Autodesk Inventor part; units mm, degrees
ref_plane "Work Plane1" through (29, 0, 0) normal (0, -1, 0) x (1, 0, 0)
ref_plane "YZ Plane" through (0, 0, 0) normal (1, 0, 0) x (0, 1, 0)
ref_plane "XZ Plane" through (0, 0, 0) normal (0, 1, 0) x (-1, 0, 0)
sketch "Sketch1" plane through (0, 0, 0) normal (0, 0, 1) x (1, 0, 0)
  line L0 (-1.1667, 0) -> (80, 0)
  line L1 (80, 0) -> (80, 2.5)
  line L2 (80, 2.5) -> (58, 2.5)
  line L3 (58, 2.5) -> (57.5091, 2.5)
  line L4 (57.5091, 2.5) -> (0, 2.5)
  line L5 (0, 2.5) -> (0, 4.25)
  line L6 (0, 4.25) -> (-5, 4.25)
  line L7 (-5, 4.25) -> (-5, 2.3094)
  line L8 (-5, 2.3094) -> (-2.5, 2.3094)
  line L9 (-2.5, 2.3094) -> (-1.1667, 0)
  line L10 (-16, 0) -> (61, 0)
  line L11 (0, -0.85) -> (0, 5.1)
  line L12 (58, 2.5) -> (0, 2.5) construction
  dimension "d1" = 22
  dimension "d2" = 0.4909
  dimension "d3" = 5
  dimension "d4" = 2.5
  dimension "d5" = 60
  dimension "d6" = 5
  dimension "d7" = 5
  dimension "d8" = 4.6188
  dimension "d9" = 8.5
  dimension "d26" = 80
revolve "Body" add sketch "Sketch1" angle 360 about axis through (-1.1667, 0, 0) along (1, 0, 0)
sketch "Sketch2" plane through (-5, 0, 0) normal (-1, 0, 0) x (0, 0, 1)
  circle A0 centre (0, 0) radius 2.3094
  line L0 (0, -5.95) -> (0, 5.95)
  line L1 (-5.95, 0) -> (5.95, 0)
  line L2 (2.3094, 0) -> (1.1547, -2)
  line L3 (1.1547, -2) -> (-1.1547, -2)
  line L4 (-1.1547, -2) -> (-2.3094, 0)
  line L5 (-2.3094, 0) -> (-1.1547, 2)
  line L6 (-1.1547, 2) -> (1.1547, 2)
  line L7 (1.1547, 2) -> (2.3094, 0)
extrude "Slot" add sketch "Sketch2" against normal up to next contours L7 A0 | A0 L2 | L6 L0 A0 | A0 L0 L3 | L0 L6 A0 | A0 L3 L0 | L4 A0 | A0 L5
fillet "Fillet1" radius 0.5 1 edges at (-5, -4.25, 0)
thread "Thread"
chamfer "Chamfer1" distance 0.4908 distance2 0.4908 1 edges at (80, -2.5, 0) measured on face at (80, 0.2278, 0.5045)
ref_plane "Work Plane1" through (29, 0, 0) normal (0, -1, 0) x (1, 0, 0)
fillet "Fillet2" radius 0.2 1 edges at (0, -2.5, 0)
equation "\"d30\" = R"
equation "\"d17\" = RR"
equation "\"d13\" = GEL"
equation "\"d15\" = -0.5 * SPD + 0.5 * GD"
equation "\"d16\" = GUL"
equation "\"d1\" = GEL"
equation "\"d3\" = KOH"
equation "\"d4\" = INTI"
equation "\"d6\" = GD"
equation "\"d7\" = BDM"
equation "\"d8\" = 1.1547 * SW"
equation "\"d9\" = KOD"
equation "\"d26\" = NLG"
equation "\"GD\" = NND"
equation "\"NLG\" = 80"
equation "\"GEL\" = 22"
equation "\"KOD\" = 8.5"
equation "\"KOH\" = 5"
equation "\"INTI\" = 2.5"
equation "\"GAL\" = 0.61345 * PTC"
equation "\"GUL\" = 0.61345 * PTC"
equation "\"BDM\" = NND"
equation "\"SW\" = 4"
equation "\"RR\" = 0.5"
equation "\"SPD\" = NND - 1.2269 * PTC"
equation "\"R\" = 0.2"
equation "\"TOA\" = 30deg"
equation "\"GD1\" = THREADDIA - 1.2269 * PTC"
equation "\"THREADDIA\" = 5"
equation "\"FAWI\" = 45deg"
equation "\"ANG\" = 120deg"
equation "\"PTC\" = 0.8"
equation "\"NND\" = 5"
equation "\"E0\" = 1.155 * SW"
properties material "Steel, Mild"
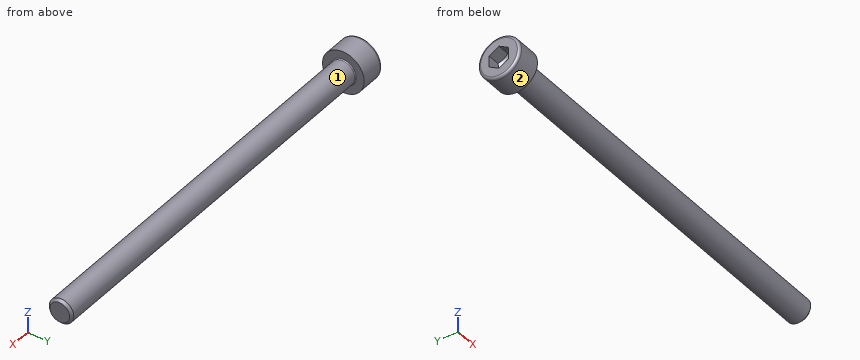
The listing builds one solid part. Answer for the finished solid, in the listing's coordinates (mm). Face numbers are marked on the shaded views. A direction names the side the tool comes from. Give positions to 0.01 mm unless a question says otherwise; leave off trailing zeros. Write each loop counter-clockwise with the first axis right and the second up, starting at its lowest first coordinate (ties: lowest second). Pieces come first, ordered by that corner, then holes. Notation, with made-up numbers: M 36,66.5 L 80,66.5 A35 ccw 80,103.5 Z; hole C -34.75,21 d1. An arc over 180 degrees is marked long. Write each question's results on one line, items separated by ' | '.
Q1. Section A-A, the plane x = 50 is taken. Write down the section's boundary in (y, z).
Output values:
outline: C 0,0 d5
Q2. Flat-ended cylindrical pins translate along their axes: P1, Ø1, axis at x = 32, z = 2.5, coming from the +Y side; P2, Ø5, axis at x = 10.5, z = -1, coming from the -Y side; P3, Ø0.7, axis at x = -3.5, z = 0.5, coming from the +Y side; P4, Ø1, axis at y = 3.5, z = -2, coming from the -X side. Find the tip coordinate at first contact, or state that the pin passes through.
Output values:
P1: y = 1.5 | P2: y = -2.5 | P3: y = 4.25 | P4: x = -5
Q3. A tool of negligible diameter and unlimited length cuts with its end or side. For the marked faces 1 and 2, from which of +Z, -Z, +X, -X, +Y, -Y can it reach the whole face along a straight path? Write none if from no direction.
Output values:
face 1: +X | face 2: +X, -X
Q4. Consider L1, parallel to X at y = 1.5, z = -3.5; L2, parallel to Z at x = 25, y = 0.25; L3, parallel to Y at x = 53.5, z = -1. Determine where each line is inside the solid, lowest interval first. Write a range as from..to.
Output values:
L1: -5..0 | L2: -2.49..2.49 | L3: -2.29..2.29
